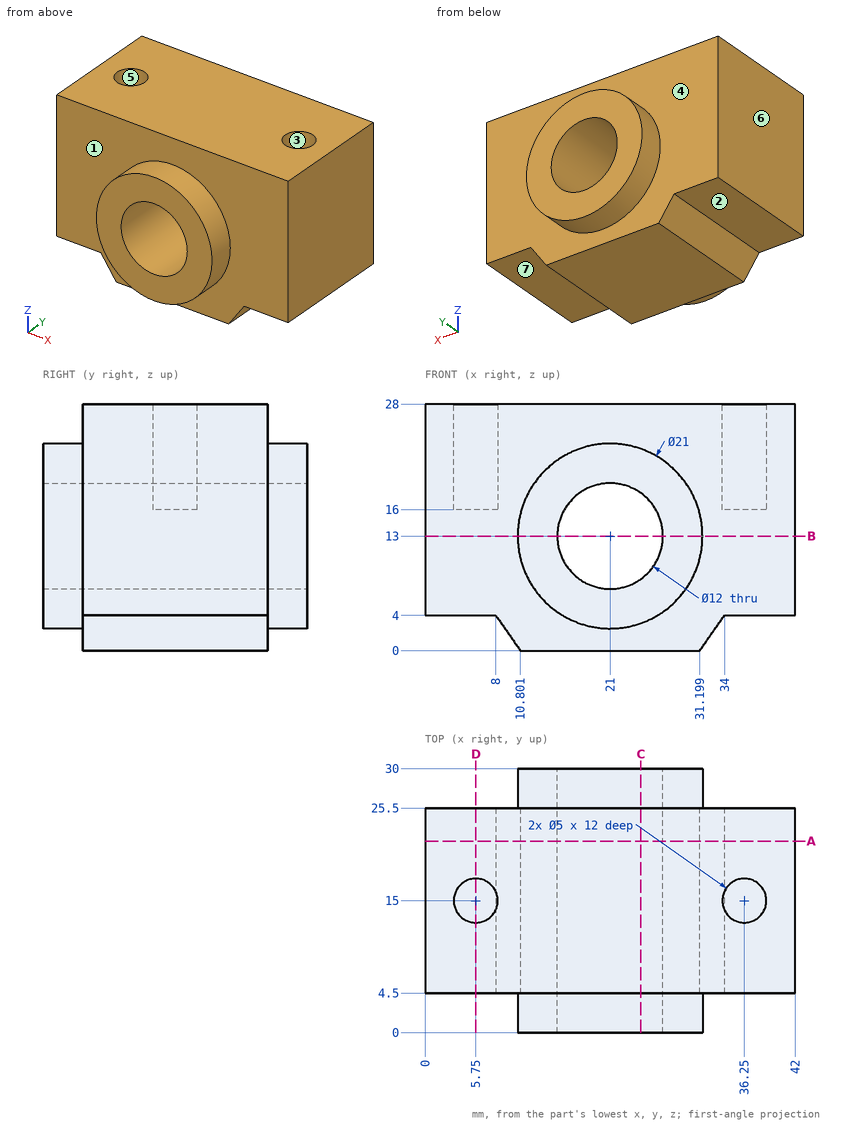
Geometry: see drawing. Coordinates: mm, zero at the bounding-box minimum. A direction names the side the tool comes from. Give positions to 0.01 mm unless a question says otherwise; leave off trailing zeros. Loops run counter-clockwise (first coordinate to the right, second up) from the corner with the lowest first, then second, coordinate; pieces in that order, holes last. Notation, with made-up numbers: M 16.25,-36 L 56.25,-36 A30 ccw 56.25,1 Z; hole C 53,10.5 d5. An arc over 180 degrees is marked long. Use one line per item in the form item = value.
1. First-contact query: pin 1 (1.5 mm diameter, centred on y = 26.5, z = 21, fed in from -X) (1 decimal); pin 2 (4 mm diameter, centred on x = 39, y = 18.5, fed in from -Z); pin 3 (4 mm diameter, centred on x = 6, z = 5.5, fed in from -Y). Flat tips, straight axial feed; report the tip coordinate or a pass-through.
Numbers:
pin_1 = 13.4
pin_2 = 4
pin_3 = 4.5
2. Section query C-C, the plane x = 24.5. Return the cut outline in (y, z), and give its area (3 significant figures).
Numbers:
outline = M 0,3.1 L 4.5,3.1 L 4.5,0 L 25.5,0 L 25.5,3.1 L 30,3.1 L 30,8.13 L 0,8.13 Z; M 0,17.87 L 30,17.87 L 30,22.9 L 25.5,22.9 L 25.5,28 L 4.5,28 L 4.5,22.9 L 0,22.9 Z
area = 474 mm²
3. Section query D-D, the plane x = 5.75. Return the cut outline in (y, z), and give its area (3 significant figures).
Numbers:
outline = M 4.5,4 L 25.5,4 L 25.5,28 L 17.5,28 L 17.5,16 L 12.5,16 L 12.5,28 L 4.5,28 Z
area = 444 mm²
4. Section query B-B, the plane z = 13. Return the cut outline in (x, y).
Numbers:
outline = M 0,4.5 L 10.5,4.5 L 10.5,0 L 15,0 L 15,30 L 10.5,30 L 10.5,25.5 L 0,25.5 Z; M 27,0 L 31.5,0 L 31.5,4.5 L 42,4.5 L 42,25.5 L 31.5,25.5 L 31.5,30 L 27,30 Z
5. Line query: L1, parallel to Y at x = 36.25, z = 19.5; L2, parallel to Z at x = 21, y = 11; L3, parallel to X at y = 16.75, z = 18 (1 decimal). Output: solid intervals per line, ascending.
Numbers:
L1 = 4.5 to 12.5, 17.5 to 25.5
L2 = 0 to 7, 19 to 28
L3 = 0 to 4, 7.5 to 17.7, 24.3 to 34.5, 38 to 42
6. Reachability of the marked faces 1, 2, 3 and 4 from +Z, -Z, +X, -X, +Y, -Y: full face, straight path, thin tool, end or side. Return the list, or none.
Numbers:
face_1 = -Y
face_2 = -Z, -X, +Y, -Y
face_3 = +Z
face_4 = +Y
7. Section query A-A, the plane y = 21.75. Return the cut outline in (x, z), and give its area (3 significant figures).
Numbers:
outline = M 0,4 L 8,4 L 10.8,0 L 31.2,0 L 34,4 L 42,4 L 42,28 L 0,28 Z; hole C 21,13 d12
area = 988 mm²
8. Pull-direction query (X, two-part tool) for the marked faces 5, 6 and 7; classes: released by +X, released by -X, zero draft, split by the parting line, or undercut.
Numbers:
face_5 = undercut
face_6 = released by -X
face_7 = zero draft
